Geometry: final body of the model. Coordinates: model frame, mm. A direction names the side the tool comes from. Give positions to 0.01 mm unless a question says otherwise; leave off trailing zeros. Loops run counter-clockwise (first coordinate to the right, second up) from the corner with the lowest first, then second, coordinate; pieces in that order, holes last. Notation, with made-up numbers: (35.5, 24.5) - (93.5, 24.5) arc R26 cw to (93.5, 58.5) - close; hole circle Ø10 at (0, -12). An arc over 180 degrees is marked (long way). Use one line per item in the form item = value.
```python
from build123d import *

# Parameters (mm, degrees)
SKETCH2_R               = 7.5
SKETCH2_R_2             = 3
BOSS_EXTRUDE1_DEPTH     = 10
SKETCH3_R               = 3
CUT_EXTRUDE1_DEPTH      = 8.5
CUT_EXTRUDE1_DEPTH_BACK = 8.5
SKETCH3_5_R             = 4.121610416
SKETCH3_5_R_2           = 1.5
BOSS_EXTRUDE6_DEPTH     = 6
BOSS_EXTRUDE7_DEPTH     = 10
SKETCH5_R               = 3
CUT_EXTRUDE3_DEPTH      = 10
SKETCH6_R               = 4.365
BOSS_EXTRUDE8_DEPTH     = 10


with BuildPart() as part:
    # Sketch2 → Boss-Extrude1 (new body)
    with BuildSketch(Plane.XY):
        Circle(SKETCH2_R)
        Circle(SKETCH2_R_2, mode=Mode.SUBTRACT)
    extrude(amount=BOSS_EXTRUDE1_DEPTH)

    # Sketch3 → Cut-Extrude1 (cut, two sides)
    with BuildSketch(Plane(origin=(0, 0, 0), x_dir=(0, -1, 0), z_dir=(1, 0, 0))) as cut_extrude1_sk:
        with Locations((0, -5)):
            Circle(SKETCH3_R)
    extrude(amount=CUT_EXTRUDE1_DEPTH, mode=Mode.SUBTRACT)
    extrude(cut_extrude1_sk.sketch, amount=-CUT_EXTRUDE1_DEPTH_BACK, mode=Mode.SUBTRACT)

    # Sketch3<5> → Boss-Extrude6 (add, symmetric)
    with BuildSketch(Plane(origin=(0, 0, 0), x_dir=(0, -1, 0), z_dir=(1, 0, 0))):
        with Locations((0, -5)):
            Circle(SKETCH3_5_R)
        with Locations((0, -5)):
            Circle(SKETCH3_5_R_2, mode=Mode.SUBTRACT)
    extrude(amount=BOSS_EXTRUDE6_DEPTH, both=True)

    # Sketch4 → Boss-Extrude7 (add)
    with BuildSketch(Plane.XY.offset(10)):
        with BuildLine():
            ThreePointArc((-1.425, 4.125845368), (-4.365, 0), (-1.425, -4.125845368))
            Line((-1.425, -4.125845368), (-1.425, -2.639957386))
            ThreePointArc((-1.425, -2.639957386), (-3, 0), (-1.425, 2.639957386))
            Line((-1.425, 2.639957386), (-1.425, 4.125845368))
        make_face()
        with BuildLine():
            Line((-1.425, -2.639957386), (-1.425, -4.125845368))
            ThreePointArc((-1.425, -4.125845368), (0, -4.365), (1.425, -4.125845368))
            Line((1.425, -4.125845368), (1.425, -2.639957386))
            ThreePointArc((1.425, -2.639957386), (0, -3), (-1.425, -2.639957386))
        make_face()
        with BuildLine():
            ThreePointArc((1.425, 4.125845368), (0, 4.365), (-1.425, 4.125845368))
            Line((-1.425, 4.125845368), (-1.425, 2.639957386))
            ThreePointArc((-1.425, 2.639957386), (0, 3), (1.425, 2.639957386))
            Line((1.425, 2.639957386), (1.425, 4.125845368))
        make_face()
        with BuildLine():
            Line((-1.425, 5.9), (-1.425, 4.125845368))
            ThreePointArc((-1.425, 4.125845368), (0, 4.365), (1.425, 4.125845368))
            Line((1.425, 4.125845368), (1.425, 5.9))
            Line((1.425, 5.9), (-1.425, 5.9))
        make_face()
        with BuildLine():
            Line((1.425, -2.639957386), (1.425, -4.125845368))
            ThreePointArc((1.425, -4.125845368), (3.554810122, -2.533090997), (4.365, 0))
            ThreePointArc((4.365, 0), (3.554810122, 2.533090997), (1.425, 4.125845368))
            Line((1.425, 4.125845368), (1.425, 2.639957386))
            ThreePointArc((1.425, 2.639957386), (2.576334606, 1.537042615), (3, 0))
            ThreePointArc((3, 0), (2.576334606, -1.537042615), (1.425, -2.639957386))
        make_face()
        with BuildLine():
            ThreePointArc((-1.425, 2.639957386), (-3, 0), (-1.425, -2.639957386))
            Line((-1.425, -2.639957386), (-1.425, 2.639957386))
        make_face()
        with BuildLine():
            Line((-1.425, 2.639957386), (-1.425, -2.639957386))
            ThreePointArc((-1.425, -2.639957386), (0, -3), (1.425, -2.639957386))
            Line((1.425, -2.639957386), (1.425, 2.639957386))
            ThreePointArc((1.425, 2.639957386), (0, 3), (-1.425, 2.639957386))
        make_face()
        with BuildLine():
            Line((1.425, 2.639957386), (1.425, -2.639957386))
            ThreePointArc((1.425, -2.639957386), (2.576334606, -1.537042615), (3, 0))
            ThreePointArc((3, 0), (2.576334606, 1.537042615), (1.425, 2.639957386))
        make_face()
    extrude(amount=BOSS_EXTRUDE7_DEPTH)

    # Sketch5 → Cut-Extrude3 (cut)
    with BuildSketch(Plane(origin=(0, 0, 0), x_dir=(-1, 0, 0), z_dir=(0, 0, -1))):
        Circle(SKETCH5_R)
    extrude(amount=-CUT_EXTRUDE3_DEPTH, mode=Mode.SUBTRACT)

    # Sketch6 → Boss-Extrude8 (add)
    with BuildSketch(Plane.XY.offset(20)):
        Circle(SKETCH6_R)
    extrude(amount=BOSS_EXTRUDE8_DEPTH)


solid = part.part
```
(1) Material intervals for L1, parallel to X at y = 0, z = 0.9; L2, parallel to Z at x = 5.5, y = -3, sorted ascending. Write a range as from..to.
Solution:
L1 = -7.5..-3, 3..7.5
L2 = 0..10
(2) Cut plane D-D (z = 16.5). Return the cut outline in (x, y) (3 decimals).
Solution:
outline = (-1.425, 4.126) arc R4.365 ccw (long way) to (1.425, 4.126) - (1.425, 5.9) - (-1.425, 5.9) - close
(3) Access query for faces 1 (the face through (-6.57, -2.86, 4.1)), 2 (the face through (6, -1.3, 6.3)), 3 (the face through (0, 5.9, 15)), 4 (the face through (1.425, 5, 15)), 5 (the face through (0, 0, 10)). Directions: +Z, -Z, +X, -X, +Y, -Y. A direction counts if a zero-diameter tool reaches every point of the face in a straight line with its end or side. Return the directions, or none.
Solution:
face_1 = -X
face_2 = +X
face_3 = +Z, +X, -X, +Y
face_4 = +Z, +X, +Y
face_5 = -Z
(4) Cut plane C-C (x = 0). Return the cut outline in (y, z) (3 decimals), plus the area to 3 significant figures.
Solution:
outline = (-7.5, 0) - (-3, 0) - (-3, 10) - (3, 10) - (3, 0) - (7.5, 0) - (7.5, 10) - (5.9, 10) - (5.9, 20) - (4.365, 20) - (4.365, 30) - (-4.365, 30) - (-4.365, 10) - (-7.5, 10) - close
area = 280 mm2
(5) Cut plane A-A (y = 0.75). Return the cut outline in (x, z), plus the area to 3 significant figures.
Solution:
outline = (-7.46, 0) - (-2.9, 0) - (-2.9, 3.7) - (-6, 3.7) - (-6, 2.1) - (-7.46, 2.1) - close; (-7.46, 7.9) - (-6, 7.9) - (-6, 6.3) - (-2.9, 6.3) - (-2.9, 10) - (2.9, 10) - (2.9, 6.3) - (6, 6.3) - (6, 7.9) - (7.46, 7.9) - (7.46, 10) - (4.3, 10) - (4.3, 30) - (-4.3, 30) - (-4.3, 10) - (-7.46, 10) - close; (2.9, 0) - (7.46, 0) - (7.46, 2.1) - (6, 2.1) - (6, 3.7) - (2.9, 3.7) - close
area = 230 mm2
(6) Pull-direction query (Z, two-part tool) for faces 6 (the face through (-1.425, 5, 15)), 7 (the face through (0, 0, 30)), 8 (the face through (-6, -1.3, 6.3)); classes: released by +Z, released by -Z, zero draft, split by the parting line, or undercut.
Solution:
face_6 = zero draft
face_7 = released by +Z
face_8 = undercut
(7) Pin query (flat end, axial travel): P1, Ø1, axis at x = -2, z = 11.5, coming from the +Y side; P2, Ø0.5, axis at y = 5, z = 15, coming from the -X side (3 decimals); P3, Ø2.5, axis at y = 0, z = 5, coming from the +X side; P4, Ø6, axis at x = -4, z = 22.5, coming from the -Y side. Return the tip coordinate at first contact, or that it passes through.
Solution:
P1 = 4.1
P2 = -1.425
P3 = through
P4 = -4.25
(8) Cut plane B-B (z = 5). Return the cut outline in (x, y).
Solution:
outline = (-6.87, -3) arc R7.5 ccw to (6.87, -3) - (6, -3) - (6, -1.5) - (2.6, -1.5) arc R3 cw to (-2.6, -1.5) - (-6, -1.5) - (-6, -3) - close; (-6.87, 3) - (-6, 3) - (-6, 1.5) - (-2.6, 1.5) arc R3 cw to (2.6, 1.5) - (6, 1.5) - (6, 3) - (6.87, 3) arc R7.5 ccw to start
